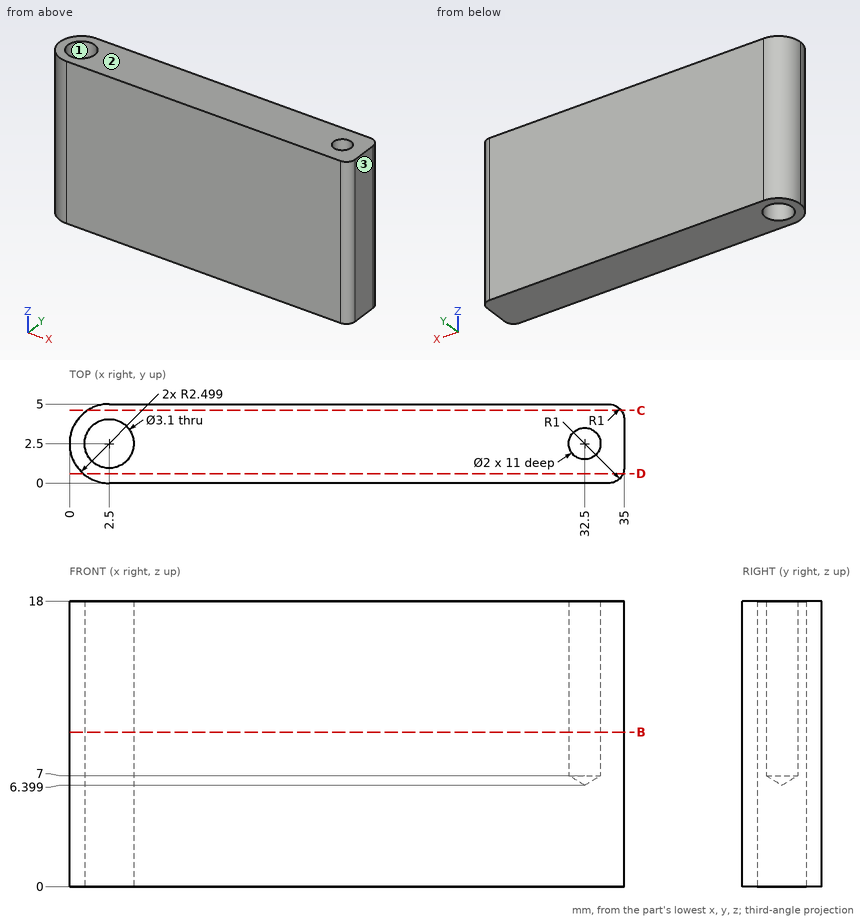
Design review of the part shown in the three views and the two pictorial views. Dimensions are in mm from the part's minimum x, y and z. Round coordinates to 2 decimals unless told otherwise and drop trailing zeros. Order: outer loops, then holes, each group sorted by start corner. A loop starts at its lowest first (then second) coordinate and runs counter-clockwise, first axis right, second up. Notation, with made-up numbers: (-6, 82) - (32, 82) arc R24 ccw to (32, 117) - close; hole circle Ø1 at (4, 23.5). An arc over 180 degrees is marked (long way). Answer in a Markdown table with one row per item.
(1) Take a section at D-D on y = 0.6. Write out the cut boundary in (x, z) (1 decimal), plus the area to 3 significant figures.
Result set:
| item | result |
|---|---|
| outline | (0.9, 0) - (34.9, 0) - (34.9, 18) - (0.9, 18) - close |
| area | 613 mm2 |
(2) Take a section at C-C on y = 4.6. Write out the cut boundary in (x, z).
Result set:
| item | result |
|---|---|
| outline | (1.14, 0) - (34.8, 0) - (34.8, 18) - (1.14, 18) - close |
(3) Mouldability with a two-part tool opening along X and no side actions: class the marked faces 1, 2 and 3 as released by +X, released by -X, zero draft, split by the parting line, or undercut.
Result set:
| item | result |
|---|---|
| face 1 | undercut |
| face 2 | zero draft |
| face 3 | released by +X |
(4) For line 1 (X direction, y = 2.5, z = 12.5); line 2 (Y direction, x = 32.5, z = 14); line 3 (Y direction, x = 2.5, z = 11), list the stretches that pass through material, from the lowest coordinate up. Write a range as from..to.
Result set:
| item | result |
|---|---|
| line 1 | x = 0..0.95, 4.05..31.5, 33.5..35 |
| line 2 | y = 0..1.5, 3.5..5 |
| line 3 | y = 0..0.95, 4.05..5 |
(5) Take a section at B-B on z = 9.75. Count the separate pieces of the cut face and the enclosed holes in it, plus the area to 3 significant figures.
Result set:
| item | result |
|---|---|
| separate pieces | 1 |
| enclosed holes | 2 |
| area | 161 mm2 |
